Could you check a few things on this model? Use its own coordinates, in mm. Round coordinates to 2 decimals unless told otherwise and drop trailing zeros. Loops run counter-clockwise (first coordinate to the right, second up) from the corner with the lowest first, then second, coordinate; pieces in that order, holes last. Notation, with made-up numbers: (55, 27.5) -> (76, 27.5) arc R13 ccw to (76, 42.5) -> close; hole circle Ø3 at (71.25, -18). An arc over 180 degrees is marked (long way). Write each question's results on one line, items separated by ' | '. Start each with the question number.
1) We'd pull the mould along Y, two halves only. Please class faces 1 (the flat face through (-0.1, -8.05, 0.5)), 2 (the flat face through (-8.1, -0.1, 0.5)), 3 (the cylindrical face through (-7.66, 3.435, 0.493)): pulls with the +Y half, pulls with the -Y half, needs draft (parallel to the pull), parting line crosses it, or undercut.
2) Imagine slicing it at B-B, the plane z = 0.8. Give the number of separate pieces and of enclosed holes in the cut face, plus the area to 3 significant figures.
3) If I drill on probe 1 along X at (y, z) = (1, 0.6); probe 2 along X at (y, z) = (-6.5, 0.55), over which ranges is the centre line in solid material (lowest first)?
4) Imagine slicing it at A-A, the plane y = -4.95. List the corners of the cut face in (x, z) for me, plus the area to 3 significant figures.
from build123d import *

# Parameters (mm, degrees)
CROQUIS1_W              = 16.2
CROQUIS1_H              = 16.1
CROQUIS1_R              = 0.57
SALIENTE_EXTRUIR1_DEPTH = 1


with BuildPart() as part:
    # Croquis1 → Saliente-Extruir1 (new body)
    with BuildSketch(Plane.XY):
        Rectangle(CROQUIS1_W, CROQUIS1_H)
        with Locations((-7.24, 7.05)):
            Circle(CROQUIS1_R, mode=Mode.SUBTRACT)
        with Locations((-7.24, 5.05)):
            Circle(CROQUIS1_R, mode=Mode.SUBTRACT)
        with Locations((-7.24, 3.05)):
            Circle(CROQUIS1_R, mode=Mode.SUBTRACT)
        with Locations((-7.24, 1.05)):
            Circle(CROQUIS1_R, mode=Mode.SUBTRACT)
        with Locations((-7.24, -0.95)):
            Circle(CROQUIS1_R, mode=Mode.SUBTRACT)
        with Locations((-7.24, -2.95)):
            Circle(CROQUIS1_R, mode=Mode.SUBTRACT)
        with Locations((-7.24, -4.95)):
            Circle(CROQUIS1_R, mode=Mode.SUBTRACT)
        with Locations((-7.24, -6.95)):
            Circle(CROQUIS1_R, mode=Mode.SUBTRACT)
        with Locations(Location((7.24, -6.95, 0), (0, 0, 180))):
            Circle(CROQUIS1_R, mode=Mode.SUBTRACT)
        with Locations(Location((7.24, -4.95, 0), (0, 0, 180))):
            Circle(CROQUIS1_R, mode=Mode.SUBTRACT)
        with Locations(Location((7.24, -2.95, 0), (0, 0, 180))):
            Circle(CROQUIS1_R, mode=Mode.SUBTRACT)
        with Locations(Location((7.24, -0.95, 0), (0, 0, 180))):
            Circle(CROQUIS1_R, mode=Mode.SUBTRACT)
        with Locations(Location((7.24, 1.05, 0), (0, 0, 180))):
            Circle(CROQUIS1_R, mode=Mode.SUBTRACT)
        with Locations(Location((7.24, 3.05, 0), (0, 0, 180))):
            Circle(CROQUIS1_R, mode=Mode.SUBTRACT)
        with Locations(Location((7.24, 5.05, 0), (0, 0, 180))):
            Circle(CROQUIS1_R, mode=Mode.SUBTRACT)
        with Locations(Location((7.24, 7.05, 0), (0, 0, 180))):
            Circle(CROQUIS1_R, mode=Mode.SUBTRACT)
    extrude(amount=SALIENTE_EXTRUIR1_DEPTH)


solid = part.part
Checked values:
1) face 1: pulls with the -Y half | face 2: needs draft | face 3: undercut
2) separate pieces: 1 | enclosed holes: 16 | area: 244 mm^2
3) probe 1: -8.1 to -7.81, -6.67 to 6.67, 7.81 to 8.1 | probe 2: -8.1 to -7.59, -6.89 to 6.89, 7.59 to 8.1
4) outline: (-8.1, 0) -> (-7.81, 0) -> (-7.81, 1) -> (-8.1, 1) -> close; (-6.67, 0) -> (6.67, 0) -> (6.67, 1) -> (-6.67, 1) -> close; (7.81, 0) -> (8.1, 0) -> (8.1, 1) -> (7.81, 1) -> close | area: 13.9 mm^2
